Can you work these out from the model? Positions are in its coordinate system, mm. Coordinates: 2 decimals unless noted, no trailing zeros. Order: outer loops, then holes, each group sorted by start corner. A loop starts at its lowest first (then second) coordinate and runs counter-clockwise, first axis right, second up. Notation, with made-up numbers: (-15.5, -22) -> (-2.5, -22) arc R24 ccw to (-2.5, 1) -> close; hole circle Ø11 at (63, -25). An arc over 180 degrees is marked (long way). Answer as CSV lines item,"result".
from build123d import *

# Parameters (mm, degrees)
SKETCH1_R           = 5
BOSS_EXTRUDE1_DEPTH = 10
SKETCH2_W           = 30
SKETCH2_H           = 30
BOSS_EXTRUDE2_DEPTH = 10
BOSS_EXTRUDE3_START = -20
SKETCH1_2_R         = 5
BOSS_EXTRUDE3_DEPTH = 10
SKETCH3_W           = 500
SKETCH3_H           = 400
BOSS_EXTRUDE4_DEPTH = 10


with BuildPart() as part:
    # Sketch1 → Boss-Extrude1 (new body)
    with BuildSketch(Plane(origin=(0, 0, 0), x_dir=(1, 0, 0), z_dir=(0, 1, 0))):
        with BuildLine():
            Line((0, 15), (-20, 15))
            Line((-20, 15), (-20, -15))
            Line((-20, -15), (0, -15))
            ThreePointArc((0, -15), (15, 0), (0, 15))
        make_face()
        with Locations(Location((0, 0, 0), (0, 0, 270))):
            Circle(SKETCH1_R, mode=Mode.SUBTRACT)
    extrude(amount=-BOSS_EXTRUDE1_DEPTH)

    # Sketch2 → Boss-Extrude2 (add)
    with BuildSketch(Plane.ZY.offset(20)):
        with Locations((0, -15)):
            Rectangle(SKETCH2_W, SKETCH2_H)
    extrude(amount=BOSS_EXTRUDE2_DEPTH)

    # Sketch1_2 → Boss-Extrude3 (add)
    with BuildSketch(Plane(origin=(0, 0, 0), x_dir=(1, 0, 0), z_dir=(0, 1, 0)).offset(BOSS_EXTRUDE3_START)):
        with BuildLine():
            Line((0, 15), (-20, 15))
            Line((-20, 15), (-20, -15))
            Line((-20, -15), (0, -15))
            ThreePointArc((0, -15), (15, 0), (0, 15))
        make_face()
        with Locations(Location((0, 0, 0), (0, 0, 270))):
            Circle(SKETCH1_2_R, mode=Mode.SUBTRACT)
    extrude(amount=-BOSS_EXTRUDE3_DEPTH)

    # Sketch3 → Boss-Extrude4 (add)
    with BuildSketch(Plane.XZ.offset(30)):
        with Locations((220, 0)):
            Rectangle(SKETCH3_W, SKETCH3_H)
    extrude(amount=BOSS_EXTRUDE4_DEPTH)


solid = part.part
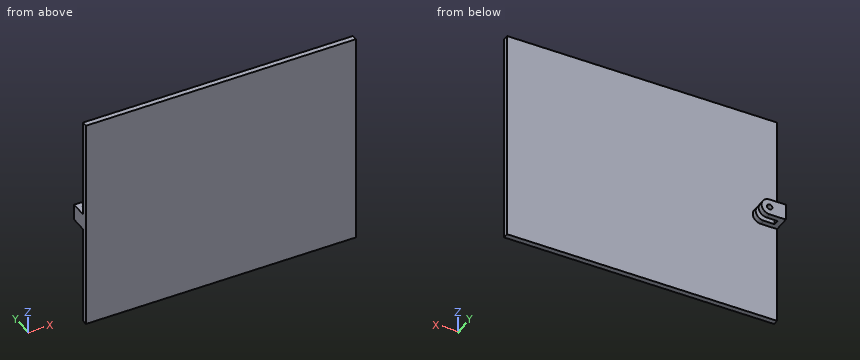
Q1. For P1, Ø13, axis at x = 0, z = 0, coming from the +Y side; P2, Ø1, axis at x = 137, z = -138, coming from the +Y side; P3, Ø11, axis at y = -14.5, z = -7.5, coming from the +X side; P4, Ø24, axis at x = -7.5, y = -9.5, coming from the -Z side, each with a flat end and sliding along its axis, tell me the tip position at first contact or that it passes through.
Solution:
P1,"y = 0"
P2,"y = -30"
P3,"x = 14.36"
P4,"z = -15"
Q2. Imagine slicing it at A-A (z = 32). List the corners of the cut face in (x, y) for me.
Solution:
outline,"(-30, -40) -> (470, -40) -> (470, -30) -> (-30, -30) -> close"
Q3. Imagine slicing it at B-B (x = 217). List the corners of the cut face in (y, z) for me.
Solution:
outline,"(-40, -200) -> (-30, -200) -> (-30, 200) -> (-40, 200) -> close"
Q4. If I drill on line 1 (X direction, y = -22.75, z = 0); line 2 (Y direction, x = 198, z = -42.5), over which ranges is the centre line in solid material (lowest first)?
Solution:
line 1,"-30 to -5, 5 to 15"
line 2,"-40 to -30"
